CAD build for the part. Positions are in the model's coordinates, mm. A direction names the side the tool comes from. Round coordinates to 2 decimals unless told otherwise and drop trailing zeros. Order: outer loops, then holes, each group sorted by start corner. A loop starts at its lowest first (then second) coordinate and runs counter-clockwise, first axis right, second up. Notation, with made-up numbers: (36, -26) - (43, -26) arc R20 ccw to (43, -18) - close; hole circle Ø4 at (28, -24.75). An arc over 180 degrees is marked (long way). Write item = value, one per line.
from build123d import *

# Parameters (mm, degrees)
ESBO_O1_W                = 13.25
ESBO_O1_H                = 12.5
RESSALTO_EXTRUS_O1_DEPTH = 4.65
ESBO_O2_W                = 13.25
ESBO_O2_H                = 32.05
RESSALTO_EXTRUS_O2_DEPTH = 5
ESBO_O3_W                = 13.25
ESBO_O3_H                = 4.65
RESSALTO_EXTRUS_O3_DEPTH = 12.5
ESBO_O4_W                = 13.25
ESBO_O4_H                = 5
RESSALTO_EXTRUS_O4_DEPTH = 10
ESBO_O5_W                = 13.25
ESBO_O5_H                = 5
RESSALTO_EXTRUS_O5_DEPTH = 10
ESBO_O6_R                = 1.5
CORTE_EXTRUS_O1_DEPTH    = 10
ESBO_O7_R                = 1
CORTE_EXTRUS_O2_DEPTH    = 14.25
ESBO_O8_R                = 1
CORTE_EXTRUS_O3_DEPTH    = 14.25
ESBO_O9_W                = 3
ESBO_O9_H                = 10.390977072
CORTE_EXTRUS_O4_DEPTH    = 10
ESBO_O10_W               = 3
ESBO_O10_H               = 2
CORTE_EXTRUS_O5_DEPTH    = 10
FILETE1_R                = 5
FILETE2_R                = 5


with BuildPart() as part:
    # Esboço1 → Ressalto-extrusão1 (new body)
    with BuildSketch(Plane(origin=(0, 0, 0), x_dir=(1, 0, 0), z_dir=(0, 1, 0))):
        with Locations((-15.112918198, -12.411797698)):
            Rectangle(ESBO_O1_W, ESBO_O1_H)
    extrude(amount=-RESSALTO_EXTRUS_O1_DEPTH)

    # Esboço2 → Ressalto-extrusão2 (add)
    with BuildSketch(Plane(origin=(0, 0, 6.161797698), x_dir=(-1, 0, 0), z_dir=(0, 0, -1))):
        with Locations((15.112918198, -16.025)):
            Rectangle(ESBO_O2_W, ESBO_O2_H)
    extrude(amount=RESSALTO_EXTRUS_O2_DEPTH)

    # Esboço3 → Ressalto-extrusão3 (add)
    with BuildSketch(Plane.XY.offset(6.161797698)):
        with Locations((-15.112918198, -29.725)):
            Rectangle(ESBO_O3_W, ESBO_O3_H)
    extrude(amount=RESSALTO_EXTRUS_O3_DEPTH)

    # Esboço4 → Ressalto-extrusão4 (add)
    with BuildSketch(Plane(origin=(0, -32.05, 0), x_dir=(-1, 0, 0), z_dir=(0, -1, 0))):
        with Locations((15.112918198, -16.161797698)):
            Rectangle(ESBO_O4_W, ESBO_O4_H)
    extrude(amount=RESSALTO_EXTRUS_O4_DEPTH)

    # Esboço5 → Ressalto-extrusão5 (add)
    with BuildSketch(Plane(origin=(0, 0, 0), x_dir=(1, 0, 0), z_dir=(0, 1, 0))):
        with Locations((-15.112918198, -16.161797698)):
            Rectangle(ESBO_O5_W, ESBO_O5_H)
    extrude(amount=RESSALTO_EXTRUS_O5_DEPTH)

    # Esboço6 → Corte-extrusão1 (cut)
    with BuildSketch(Plane(origin=(0, 0, 13.661797698), x_dir=(-1, 0, 0), z_dir=(0, 0, -1))):
        with Locations((15.112918198, 5)):
            Circle(ESBO_O6_R)
        with Locations((15.112918198, -37.05)):
            Circle(ESBO_O6_R)
    extrude(amount=-CORTE_EXTRUS_O1_DEPTH, mode=Mode.SUBTRACT)

    # Esboço7 → Corte-extrusão2 (cut, through all)
    with BuildSketch(Plane(origin=(-8.487918198, 0, 0), x_dir=(0, 0, -1), z_dir=(1, 0, 0))):
        with Locations((-12.411797698, -2.325)):
            Circle(ESBO_O7_R)
    extrude(amount=-CORTE_EXTRUS_O2_DEPTH, mode=Mode.SUBTRACT)

    # Esboço8 → Corte-extrusão3 (cut, through all)
    with BuildSketch(Plane(origin=(-8.487918198, 0, 0), x_dir=(0, 0, -1), z_dir=(1, 0, 0))):
        with Locations((-12.411797698, -29.725)):
            Circle(ESBO_O8_R)
    extrude(amount=-CORTE_EXTRUS_O3_DEPTH, mode=Mode.SUBTRACT)

    # Esboço9 → Corte-extrusão4 (cut)
    with BuildSketch(Plane(origin=(0, 0, 0), x_dir=(1, 0, 0), z_dir=(0, 1, 0))):
        with Locations((-11.987918198, -13.466309162)):
            Rectangle(ESBO_O9_W, ESBO_O9_H)
    extrude(amount=-CORTE_EXTRUS_O4_DEPTH, mode=Mode.SUBTRACT)

    # Esboço10 → Corte-extrusão5 (cut)
    with BuildSketch(Plane(origin=(0, 0, 13.661797698), x_dir=(-1, 0, 0), z_dir=(0, 0, -1))):
        with Locations((11.987918198, 1)):
            Rectangle(ESBO_O10_W, ESBO_O10_H)
    extrude(amount=-CORTE_EXTRUS_O5_DEPTH, mode=Mode.SUBTRACT)

    # Filete1
    filete1_edges = [part.edges().sort_by_distance(p)[0] for p in [
        (-15.112918198, 0, 1.161797698),
    ]]
    fillet(filete1_edges, radius=FILETE1_R)

    # Filete2
    filete2_edges = [part.edges().sort_by_distance(p)[0] for p in [
        (-15.112918198, -32.05, 1.161797698),
    ]]
    fillet(filete2_edges, radius=FILETE2_R)


solid = part.part
(1) Tool access for faces 4 (the flat face through (-13.5, -38.1, 13.662)), 5 (the flat face through (-10.488, -2, 15)), 6 (the flat face through (-15, -27.4, 12)): list every direction of +Z, -Z, +X, -X, +Y, -Y with a clear straight run to the whole face (end or side of a thin tool).
Solved:
face_4 = -Z, +X, -X, -Y
face_5 = +Z
face_6 = +Z, +X, -X
(2) Band-saw the part on A-A on z = 15.25. List the corners of the cut face in (x, y), plus the area to 3 significant figures.
Solved:
outline = (-21.74, -42.05) - (-8.49, -42.05) - (-8.49, -27.4) - (-21.74, -27.4) - close; (-21.74, -4.65) - (-13.49, -4.65) - (-13.49, 2) - (-10.49, 2) - (-10.49, -4.65) - (-8.49, -4.65) - (-8.49, 10) - (-21.74, 10) - close; hole circle Ø3 at (-15.11, -37.05); hole circle Ø3 at (-15.11, 5)
area = 354 mm²
(3) Band-saw the part on B-B on x = -14.25. List the corners of the cut face in (y, z) (3 decimals), plus the area to 3 significant figures.
Solved:
outline = (-42.05, 13.662) - (-38.277, 13.662) - (-38.277, 18.662) - (-42.05, 18.662) - close; (-35.823, 13.662) - (-32.05, 13.662) - (-32.05, 6.162) arc R5 ccw to (-27.05, 1.162) - (-5, 1.162) arc R5 ccw to (0, 6.162) - (0, 13.662) - (3.773, 13.662) - (3.773, 18.662) - (-4.65, 18.662) - (-4.65, 6.162) - (-27.4, 6.162) - (-27.4, 18.662) - (-35.823, 18.662) - close; (6.227, 13.662) - (10, 13.662) - (10, 18.662) - (6.227, 18.662) - close; hole circle Ø2 at (-29.725, 12.412); hole circle Ø2 at (-2.325, 12.412)
area = 335 mm²
(4) Band-saw the part on C-C on y = -37.05. List the corners of the cut face in (x, z).
Solved:
outline = (-21.74, 13.66) - (-16.61, 13.66) - (-16.61, 18.66) - (-21.74, 18.66) - close; (-13.61, 13.66) - (-8.49, 13.66) - (-8.49, 18.66) - (-13.61, 18.66) - close
(5) Band-saw the part on D-D on x = -9.75. List the corners of the cut face in (y, z) (3 decimals).
Solved:
outline = (-42.05, 13.662) - (-32.05, 13.662) - (-32.05, 6.162) arc R5 ccw to (-27.05, 1.162) - (-5, 1.162) arc R5 ccw to (0, 6.162) - (0, 13.662) - (10, 13.662) - (10, 18.662) - (-4.65, 18.662) - (-4.65, 6.162) - (-27.4, 6.162) - (-27.4, 18.662) - (-42.05, 18.662) - close; hole circle Ø2 at (-29.725, 12.412); hole circle Ø2 at (-2.325, 12.412)
(6) Pull direction Y, two halves, no side cores. Call faces 1 (the flat face through (-16, 0, 10)), 2 (the flat face through (-12, -2, 8.271)), 3 (the cylindrical face through (-9.47, -2.02, 11.46)): released by +Y, released by -Y, zero draft, split by the parting line, or undercut.
Solved:
face_1 = released by +Y
face_2 = zero draft
face_3 = undercut
(7) Probe line 1 along X through (y, z) = (-3.5, 9); line 2 along Y through (x, z) = (-17, 13.5). List the from-to ranges inside material, lowest first.
Solved:
line_1 = -21.74 to -13.49, -10.49 to -8.49
line_2 = -32.05 to -27.4, -4.65 to 0
(8) Drop flat-ended pins along their axis: pin 1 (6 mm diameter, centred on x = -18, z = 9.5, fed in from -Y); pin 2 (3 mm diameter, centred on x = -10, y = -30.5, fed in from -Z); pin 3 (3.5 mm diameter, centred on x = -15.11, y = 5, fed in from -Z); pin 4 (1.8 mm diameter, centred on x = -15.11, y = -37.05, fed in from +Z). Give the stop position or say it passes through.
Solved:
pin_1 = -32.05
pin_2 = 1.56
pin_3 = 13.66
pin_4 = through
